```python
from build123d import *

# Parameters (mm, degrees)
BOSS_EXTRUDE1_DEPTH = 17.15
CUT_EXTRUDE1_DEPTH  = 69
CUT_EXTRUDE2_DEPTH  = 49.5
SKETCH4_R           = 2.875
CUT_EXTRUDE3_DEPTH  = 34.3
SKETCH5_R           = 2.5
CUT_EXTRUDE4_DEPTH  = 69
FILLET2_R           = 0.5


with BuildPart() as part:
    # Sketch1 → Boss-Extrude1 (new body, symmetric)
    with BuildSketch(Plane.XY):
        Polygon((-32.45, -6), (-32.45, 40.95), (32.45, 40.95), (32.45, -6), (34, -6), (34, 42.5), (-34, 42.5), (-34, -6), align=None)
    extrude(amount=BOSS_EXTRUDE1_DEPTH, both=True)

    # Sketch2 → Cut-Extrude1 (cut, through all)
    with BuildSketch(Plane.ZY.offset(34)):
        with BuildLine():
            Line((-5.981406604, -0.471990503), (-9.25, 40.95))
            Line((-9.25, 40.95), (-17.15, 40.95))
            Line((-17.15, 40.95), (-17.15, -6))
            Line((-17.15, -6), (0, -6))
            ThreePointArc((0, -6), (-4.07234926, -4.406355808), (-5.981406604, -0.471990503))
        make_face()
    cut_extrude1 = extrude(amount=-CUT_EXTRUDE1_DEPTH, mode=Mode.SUBTRACT)

    # Mirror1: Cut-Extrude1 across plane
    add(cut_extrude1.mirror(Plane.XY), mode=Mode.SUBTRACT)

    # Sketch3 → Cut-Extrude2 (cut, through all)
    with BuildSketch(Plane(origin=(0, 42.5, 0), x_dir=(1, 0, 0), z_dir=(0, 1, 0))):
        with BuildLine():
            Line((-32.5, -9.25), (-14.021657356, -9.875))
            ThreePointArc((-14.021657356, -9.875), (-7.898298867, -15.222988373), (0, -17.15))
            Line((0, -17.15), (-34, -17.15))
            Line((-34, -17.15), (-34, -9.25))
            Line((-34, -9.25), (-32.5, -9.25))
        make_face()
        with BuildLine():
            Line((-34, 9.25), (-34, 17.15))
            Line((-34, 17.15), (0, 17.15))
            ThreePointArc((0, 17.15), (-7.898298867, 15.222988373), (-14.021657356, 9.875))
            Line((-14.021657356, 9.875), (-32.5, 9.25))
            Line((-32.5, 9.25), (-34, 9.25))
        make_face()
    cut_extrude2 = extrude(amount=-CUT_EXTRUDE2_DEPTH, mode=Mode.SUBTRACT)

    # Mirror2: Cut-Extrude2 across plane
    add(cut_extrude2.mirror(Plane(origin=(0, 0, 0), x_dir=(0, 0, 1), z_dir=(1, 0, 0))), mode=Mode.SUBTRACT)

    # Sketch4 → Cut-Extrude3 (cut)
    with BuildSketch(Plane(origin=(0, 42.5, 0), x_dir=(1, 0, 0), z_dir=(0, 1, 0))):
        Circle(SKETCH4_R)
        with BuildLine():
            ThreePointArc((-8.485281374, 8.485281374), (-12, 0), (-8.485281374, -8.485281374))
            ThreePointArc((-8.485281374, -8.485281374), (-6.363961031, -8.485281374), (-6.363961031, -6.363961031))
            ThreePointArc((-6.363961031, -6.363961031), (-9, 0), (-6.363961031, 6.363961031))
            ThreePointArc((-6.363961031, 6.363961031), (-6.363961031, 8.485281374), (-8.485281374, 8.485281374))
        make_face()
    extrude(amount=-CUT_EXTRUDE3_DEPTH, mode=Mode.SUBTRACT)

    # Sketch5 → Cut-Extrude4 (cut, through all)
    with BuildSketch(Plane.ZY.offset(34)):
        Circle(SKETCH5_R)
    extrude(amount=-CUT_EXTRUDE4_DEPTH, mode=Mode.SUBTRACT)

    # Fillet2
    fillet2_edges = [part.edges().sort_by_distance(p)[0] for p in [
        (34, 42.5, 0),
        (32.45, 40.95, 0),
        (-32.45, 40.95, 0),
        (-34, 42.5, 0),
    ]]
    fillet(fillet2_edges, radius=FILLET2_R)


solid = part.part
```
Verification items for the finished model (mm, model axes). A direction names the side the tool comes from. Round coordinates to 2 decimals unless told otherwise and drop trailing zeros. Order: outer loops, then holes, each group sorted by start corner. A loop starts at its lowest first (then second) coordinate and runs counter-clockwise, first axis right, second up. Notation, with made-up numbers: (30, -13) - (51, -13) arc R19 cw to (51, 24) - close; hole circle Ø7 at (76, -22.75). An arc over 180 degrees is marked (long way). Use CSV: the item, a comma, the result in double quotes. Start each with the question number.
1) Access from +Z, -Z, +X, -X, +Y, -Y to the whole of each face (thin tool, end or side, straight path). Record for faces 1 (the flat face through (-33, 42, 9.25)), 2 (the flat face through (32.45, 18, 0)), 3 (the cylindrical face through (-9, 42, 0)), 4 (the flat face through (33, 42, -9.25)).
2) Section check C-C, the plane z = 5. Record the cut outline in (x, y), plus the area to 3 significant figures.
3) Section check B-B, the plane x = -10. Record the cut outline in (y, z), plus the area to 3 significant figures.
4) Section check A-A, the plane y = 11.5. Record the cut outline in (x, z).
5) Go/stop test with flat-tipped pins: P1, Ø3, axis at x = -13, z = 8.5, coming from the -Y side; P2, Ø1.6, axis at x = -33, y = 41.5, coming from the +Z side; P3, Ø0.8, axis at x = 33, y = 42, coming from the +Z side. Record where each tip stops, or that it passes through.
6) Section check D-D, the plane y = 1. Record the cut outline in (x, z), plus the area to 3 significant figures.
7) Thickness scan on L1, parallel to X at y = 42, z = 0 (3 decimals); L2, parallel to X at y = 2.5, z = 2; L3, parallel to Z at x = 0, y = 42.15 (3 decimals). Record the ranges inside material, lowest first.
8) Mould release check, pull along X, two halves, no side actions. Record for faces 5 (the flat face through (34, 18, 0)), 6 (the cylindrical face through (-6.39, 41.74, 8.51)), 7 (the flat face through (33.188, 19.949, -7.593)), 8 (the flat face through (-32.45, 22, 0)): +X half, -X half, draft (parallel to the pull), parting line (faces both ways), or undercut.
Answers:
1,face 1,"+Z, -X, +Y, -Y"
1,face 2,"+Z, -Z, -Y"
1,face 3,"+Y, -Y"
1,face 4,"-Z, +X, +Y, -Y"
2,outline,"(-34, -3.32) - (-32.45, -3.32) - (-32.45, 40.45) arc R0.5 cw to (-31.95, 40.95) - (-10.91, 40.95) - (-10.91, 42.5) - (-33.5, 42.5) arc R0.5 ccw to (-34, 42) - close; (-7.48, 40.95) - (31.95, 40.95) arc R0.5 cw to (32.45, 40.45) - (32.45, -3.32) - (34, -3.32) - (34, 42) arc R0.5 ccw to (33.5, 42.5) - (-7.48, 42.5) - close"
2,area,"237 mm²"
3,outline,"(40.95, -13.93) - (42.5, -13.93) - (42.5, -6.63) - (40.95, -6.63) - close; (40.95, 6.63) - (42.5, 6.63) - (42.5, 13.93) - (40.95, 13.93) - close"
3,area,"22.6 mm²"
4,outline,"(-34, -6.93) - (-32.45, -6.93) - (-32.45, 6.93) - (-34, 6.93) - close; (32.45, -6.93) - (34, -6.93) - (34, 6.93) - (32.45, 6.93) - close"
5,P1,"stops at y = 40.95"
5,P2,"stops at z = 9.26"
5,P3,"stops at z = 9.25"
6,outline,"(-34, -6.1) - (-32.45, -6.1) - (-32.45, -2.29) - (-34, -2.29) - close; (-34, 2.29) - (-32.45, 2.29) - (-32.45, 6.1) - (-34, 6.1) - close; (32.45, -6.1) - (34, -6.1) - (34, -2.29) - (32.45, -2.29) - close; (32.45, 2.29) - (34, 2.29) - (34, 6.1) - (32.45, 6.1) - close"
6,area,"23.6 mm²"
7,L1,"x = -34 to -12, -9 to -2.875, 2.875 to 34"
7,L2,"x = -34 to -32.45, 32.45 to 34"
7,L3,"z = -17.15 to -2.875, 2.875 to 17.15"
8,face 5,"+X half"
8,face 6,"undercut"
8,face 7,"draft"
8,face 8,"undercut"
